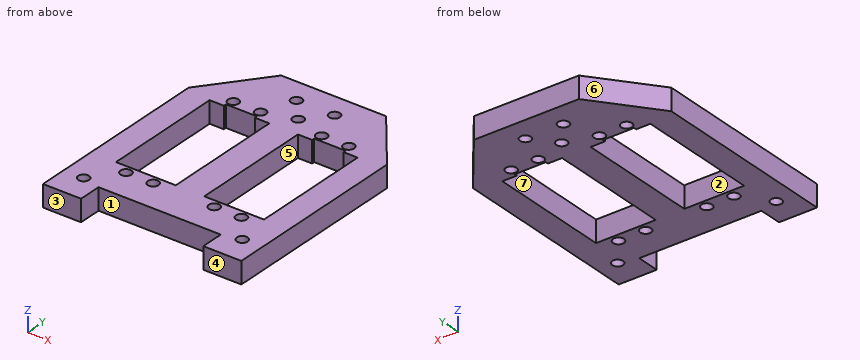
```python
from build123d import *

# Parameters (mm, degrees)
ESBO_O1_R                = 2
RESSALTO_EXTRUS_O1_DEPTH = 8


with BuildPart() as part:
    # Esboço1 → Ressalto-extrusão1 (new body)
    with BuildSketch(Plane.XY):
        Polygon((19.311716217, 17), (-19.311716217, 17), (-36.5, -5), (-36.5, -75), (-22.499999998, -75), (-22.499999998, -66.599999996), (22.499999998, -66.599999996), (22.499999998, -75), (36.5, -75), (36.5, -5), align=None)
        with Locations((-21.250245, -3.420107551)):
            Circle(ESBO_O1_R, mode=Mode.SUBTRACT)
        with Locations((-11.250245, -55.019882032)):
            Circle(ESBO_O1_R, mode=Mode.SUBTRACT)
        with Locations((11.250245, -3.420107551)):
            Circle(ESBO_O1_R, mode=Mode.SUBTRACT)
        with Locations((21.250245, -55.019882032)):
            Circle(ESBO_O1_R, mode=Mode.SUBTRACT)
        with Locations((-21.250245, -55.019882032)):
            Circle(ESBO_O1_R, mode=Mode.SUBTRACT)
        with Locations((-11.250245, -3.420107551)):
            Circle(ESBO_O1_R, mode=Mode.SUBTRACT)
        with Locations((11.250245, -55.019882032)):
            Circle(ESBO_O1_R, mode=Mode.SUBTRACT)
        with Locations((21.250245, -3.420107551)):
            Circle(ESBO_O1_R, mode=Mode.SUBTRACT)
        Circle(ESBO_O1_R, mode=Mode.SUBTRACT)
        with Locations((-7, 8.3)):
            Circle(ESBO_O1_R, mode=Mode.SUBTRACT)
        with Locations((7, 8.3)):
            Circle(ESBO_O1_R, mode=Mode.SUBTRACT)
        with Locations((-29.2, -65)):
            Circle(ESBO_O1_R, mode=Mode.SUBTRACT)
        with Locations((29.2, -65)):
            Circle(ESBO_O1_R, mode=Mode.SUBTRACT)
        Polygon((-27.250245, -29.520107551), (-27.250245, -7.020107551), (-22.000245, -7.020107551), (-22.000245, -6.020107551), (-10.500245, -6.020107551), (-10.500245, -7.020107551), (-5.250245, -7.020107551), (-5.250245, -29.520107551), (-5.250245, -52.020107551), (-27.250245, -52.020107551), align=None, mode=Mode.SUBTRACT)
        Polygon((10.500245, -7.020107551), (5.250245, -7.020107551), (5.250245, -29.520107551), (5.250245, -52.020107551), (27.250245, -52.020107551), (27.250245, -29.520107551), (27.250245, -7.020107551), (22.000245, -7.020107551), (22.000245, -6.020107551), (10.500245, -6.020107551), align=None, mode=Mode.SUBTRACT)
    extrude(amount=RESSALTO_EXTRUS_O1_DEPTH)


solid = part.part
```
The model under review builds one solid part; all positions refer to its coordinate system, in mm. Face numbers are marked on the shaded views. A direction names the side the tool comes from. Round coordinates to 2 decimals unless told otherwise and drop trailing zeros. Write each loop counter-clockwise with the first axis right and the second up, starting at its lowest first coordinate (ties: lowest second). Pieces come first, ordered by that corner, then holes. Notation, with made-up numbers: M 87.5,62.5 L 91.5,62.5 A15 cw 91.5,87.5 Z; hole C 80,-37 d11. An arc over 180 degrees is marked long. Use CSV: the item, a comma, the result in double quotes. Start each with the question number.
(1) We need section B-B, the plane x = 7. State the section outline as (y, z) points.
(2) We need section C-C, the plane y = 0. State the section outline as (x, z) points, then the cut area to 3 significant figures.
(3) We need section A-A, the plane x = 15. State the section outline as (y, z) points, then the cut area to 3 significant figures.
(4) For line 1 along X through (y, z) = (-50.5, 0.5); line 2 along Y through (x, z) = (-11, 0.5); line 3 along Y through (x, z) = (16, 6.75), list the stretches that pass through material, from the lowest coordinate up.
(5) Tool access review of the marked faces 1, 2 and 3: name each direction out of +Z, -Z, +X, -X, +Y, -Y from which nothing blocks a thin tool from reaching the whole face with its end or side.
(6) The part is to be moulded in two halves that separate along Y. For the marked faces 4, 5, 6 and 7, say which applies: +Y half, -Y half, draft (parallel to the pull), parting line (faces both ways), or undercut.
(7) We need section D-D, the plane y = -41. State the section outline as (x, z) points, then the cut area to 3 significant figures.
(8) Clearance check with a flat-ended pin moving along its axis: P1, Ø3.5, axis at x = -29.2, y = -65, coming from the -Z side. State where the tip first meets the part, or that it passes through.
Findings:
1,outline,"M -66.6,0 L -52.02,0 L -52.02,8 L -66.6,8 Z; M -7.02,0 L 6.3,0 L 6.3,8 L -7.02,8 Z; M 10.3,0 L 17,0 L 17,8 L 10.3,8 Z"
2,outline,"M -32.59,0 L -2,0 L -2,8 L -32.59,8 Z; M 2,0 L 32.59,0 L 32.59,8 L 2,8 Z"
2,area,"489 mm^2"
3,outline,"M -66.6,0 L -52.02,0 L -52.02,8 L -66.6,8 Z; M -6.02,0 L 17,0 L 17,8 L -6.02,8 Z"
3,area,"301 mm^2"
4,line 1,"-36.5 to -27.25, -5.25 to 5.25, 27.25 to 36.5"
4,line 2,"-66.6 to -57, -53.04 to -52.02, -6.02 to -5.4, -1.44 to 17"
4,line 3,"-66.6 to -52.02, -6.02 to 17"
5,face 1,"+Z, -Z, -Y"
5,face 2,"+Z, -Z"
5,face 3,"+Z, -Z, +X, -X, -Y"
6,face 4,"-Y half"
6,face 5,"undercut"
6,face 6,"+Y half"
6,face 7,"undercut"
7,outline,"M -36.5,0 L -27.25,0 L -27.25,8 L -36.5,8 Z; M -5.25,0 L 5.25,0 L 5.25,8 L -5.25,8 Z; M 27.25,0 L 36.5,0 L 36.5,8 L 27.25,8 Z"
7,area,"232 mm^2"
8,P1,"through"
